from build123d import *

# Parameters (mm, degrees)
F0_R     = 38.7
F0_R_2   = 3
F1_DEPTH = 2


# Not quite as in the source:
# - a fillet or chamfer that OpenCascade refuses, or shapes differently, is made with other operations: its cross-section is extruded or revolved along the edge and cut away or added


with BuildPart() as f1:
    # F0 (on Top) → F1 (new body)
    with BuildSketch(Plane.XY):
        Circle(F0_R)
        with Locations((0, -21.5)):
            Circle(F0_R_2, mode=Mode.SUBTRACT)
        with Locations((-21.5, 0)):
            Circle(F0_R_2, mode=Mode.SUBTRACT)
        with Locations((21.5, 0)):
            Circle(F0_R_2, mode=Mode.SUBTRACT)
        with Locations((0, 21.5)):
            Circle(F0_R_2, mode=Mode.SUBTRACT)
    extrude(amount=F1_DEPTH)

    # F2: fillet of radius 3 on 1 edges, made by hand

    # F2_s1 → F2_t2 (revolve, cut)
    with BuildSketch(Plane.XZ):
        with BuildLine():
            ThreePointArc((38.7, 2), (37.6036236828, 0.5505102572), (35.8715728753, 0))
            Line((35.8715728753, 0), (38.7, 0))
            Line((38.7, 0), (38.7, 2))
        make_face()
    revolve(axis=Axis((0, 0, 0), (0, 0, 1)), mode=Mode.SUBTRACT)


solid = f1.part
CAD build for the part. Positions are in the model's coordinates, mm. Coordinates: 2 decimals unless noted, no trailing zeros. Loops run counter-clockwise (first coordinate to the right, second up) from the corner with the lowest first, then second, coordinate; pieces in that order, holes last. Notation, with made-up numbers: (-28, 74) - (12, 74) arc R21 cw to (12, 109) - close; hole circle Ø5 at (-30.5, 40.5). An arc over 180 degrees is marked (long way). Write item = value, one per line. Start each with the question number.
Q1. Cut at A-A, the plane y = 0. List the corners of the cut face in (x, z), then the cut area to 3 significant figures.
Q2. Drill centre lines: L1, parallel to Y at x = 0, z = 0.4; L2, parallel to Y at x = 0, z = 0.6; L3, parallel to Y at x = -21.5, z = 0.55. Where is each one in solid material? Low to high.
Q3. Cut at B-B, the plane z = 0.55. List the corners of the cut face in (x, y).
Q4. Pull direction Y, two halves, no side cores. Call faces 1 (the cylindrical face through (18.5, 0.1, 1)), 2 (the flat face through (-1, 1, 0)): pulls with the +Y half, pulls with the -Y half, needs draft (parallel to the pull), parting line crosses it, or undercut.
Computed:
q1.outline = (-38.7, 2) arc R3 ccw to (-35.87, 0) - (-24.5, 0) - (-24.5, 2) - close; (-18.5, 0) - (18.5, 0) - (18.5, 2) - (-18.5, 2) - close; (24.5, 0) - (35.87, 0) arc R3 ccw to (38.7, 2) - (24.5, 2) - close
q1.area = 128 mm²
q2.L1 = -37.37 to -24.5, -18.5 to 18.5, 24.5 to 37.37
q2.L2 = -37.67 to -24.5, -18.5 to 18.5, 24.5 to 37.67
q2.L3 = -30.85 to -3, 3 to 30.85
q3.outline = circle Ø75.21 at (0, 0); hole circle Ø6 at (-21.5, 0); hole circle Ø6 at (0, -21.5); hole circle Ø6 at (0, 21.5); hole circle Ø6 at (21.5, 0)
q4.face_1 = undercut
q4.face_2 = needs draft
